Here's how the part is built. I have some questions about the finished solid (model axes, mm). A direction names the side the tool comes from. Coordinates: 2 decimals unless noted, no trailing zeros. Loops run counter-clockwise (first coordinate to the right, second up) from the corner with the lowest first, then second, coordinate; pieces in that order, holes last.
from build123d import *

# Parameters (mm, degrees)
F0_W     = 55.5101186037
F0_H     = 32.2702378035
F1_DEPTH = 40
F2_W     = 30.5438451469
F2_H     = 18.8575051725
F3_DEPTH = 20
F4_R     = 5
F5_DEPTH = 20.001
F7_R     = 3


# Not quite as in the source:
# - a feature of the source that left no trace in its solid (it failed there, or was rolled back) is left out


with BuildPart() as f1:
    # F0 (on Front) → F1 (new body)
    with BuildSketch(Plane.XZ):
        with Locations((27.7550593019, -16.1351189017)):
            Rectangle(F0_W, F0_H)
    extrude(amount=F1_DEPTH)

    # F2 (on face) → F3 (cut)
    with BuildSketch(Plane.XZ.offset(40)):
        with Locations((40.2381960303, -22.8414852172)):
            Rectangle(F2_W, F2_H)
    extrude(amount=-F3_DEPTH, mode=Mode.SUBTRACT)

    # F4 (on face) → F5 (cut, through all)
    with BuildSketch(Plane.XZ.offset(20)):
        with Locations((40.5101186037, -24.2702378035)):
            Circle(F4_R)
    extrude(amount=-F5_DEPTH, mode=Mode.SUBTRACT)

    # F7
    f7_edges = [f1.edges().sort_by_distance(p)[0] for p in [
        (24.966273, -40, -22.841485),
        (0, -40, -16.135119),
        (12.483137, -40, -32.270238),
        (40.238196, -40, -13.412733),
        (55.510119, -40, -6.706366),
        (27.755059, -40, 0),
    ]]
    fillet(f7_edges, radius=F7_R)


solid = f1.part
Q1. Suppose I cut it at D-D on z = -16.5. Write out the boundary of the cut face in (x, y), and give its area (3 significant figures).
Q2. Will these pins go through, and if not, where does the flat tip stop? P1, Ø18.5, axis at x = 37.5, y = -32, coming from the -Z side; P2, Ø9.5, axis at x = 41.5, z = -26, coming from the -Y side.
Q3. Suppose I cut it at C-C on x = 41. Write out the boundary of the cut face in (y, z), and give its area (3 significant figures).
Q4. Please list where these lines run through material, in increasing order: probe 1 along Z at (x, y) = (50.5, -34.5); probe 2 along X at (y, z) = (-24.5, -17); probe 3 along Y at (x, z) = (44.5, -17.5).
Q5. Suppose I cut it at B-B on y = -26. Write out the boundary of the cut face in (x, z).
Q6. For faces 4 (the cylindrical face through (54.61, -39.14, -6.61)), 5 (the flat face through (24.966, -29, -23)), which set-ups out of +Z, -Z, +X, -X, +Y, -Y let a thin tool reach every point of the face, with its end or its side?
Q7. Suppose I cut it at A-A on z = -23. Write out the boundary of the cut face in (x, y), and give its area (3 significant figures).
Q8. We'd pull the mould along Z, two halves only. Please class faces 1 (the cylindrical face through (36.825, -10.14, -20.891)), 2 (the flat face through (36.6, -20, -20.6)), 3 (the cylindrical face through (28.14, -39.1, -0.86)): pulls with the +Z half, pulls with the -Z half, needs draft (parallel to the pull), parting line crosses it, or undercut.
Check values:
1. outline: (0, -37) arc R3 ccw to (3, -40) - (21.97, -40) arc R3 ccw to (24.97, -37) - (24.97, -20) - (55.51, -20) - (55.51, 0) - (0, 0) - close
1. area: 1,610 mm2
2. P1: stops at z = -13.41
2. P2: stops at y = -20
3. outline: (-40, -10.41) arc R3 ccw to (-37, -13.41) - (-20, -13.41) - (-20, -19.29) - (0, -19.29) - (0, 0) - (-37, 0) arc R3 ccw to (-40, -3) - close; (-20, -32.27) - (0, -32.27) - (0, -29.25) - (-20, -29.25) - close
3. area: 711 mm2
4. probe 1: z = -13.41 to 0
4. probe 2: x = 0 to 24.97
4. probe 3: y = -20 to 0
5. outline: (0, -32.27) - (24.97, -32.27) - (24.97, -13.41) - (55.51, -13.41) - (55.51, 0) - (0, 0) - close
6. face 4: +Z, -Z, +X, -Y
6. face 5: -Z, +X, -Y
7. outline: (0, -37) arc R3 ccw to (3, -40) - (21.97, -40) arc R3 ccw to (24.97, -37) - (24.97, -20) - (35.67, -20) - (35.67, 0) - (0, 0) - close; (45.35, -20) - (55.51, -20) - (55.51, 0) - (45.35, 0) - close
7. area: 1,410 mm2
8. face 1: undercut
8. face 2: needs draft
8. face 3: pulls with the +Z half
